```python
from build123d import *

# Parameters (mm, degrees)
SKETCH_1_W          = 50
SKETCH_1_H          = 50
EXTRUDE_1_DEPTH     = 6
SKETCH_2_W          = 6
SKETCH_2_H          = 50
EXTRUDE_2_DEPTH     = 44
SKETCH_3_R          = 10
CUT_EXTRUDE_1_DEPTH = 44
SKETCH_4_R          = 2.5
CUT_EXTRUDE_2_DEPTH = 44


with BuildPart() as part:
    # ｽｹｯﾁ1 → ﾎﾞｽ - 押し出し1 (new body)
    with BuildSketch(Plane(origin=(0, 0, 0), x_dir=(1, 0, 0), z_dir=(0, 1, 0))):
        Rectangle(SKETCH_1_W, SKETCH_1_H)
    extrude(amount=EXTRUDE_1_DEPTH)

    # ｽｹｯﾁ2 → ﾎﾞｽ - 押し出し2 (add)
    with BuildSketch(Plane(origin=(0, 6, 0), x_dir=(1, 0, 0), z_dir=(0, 1, 0))):
        with Locations((22, 0)):
            Rectangle(SKETCH_2_W, SKETCH_2_H)
    extrude(amount=EXTRUDE_2_DEPTH)

    # ｽｹｯﾁ3 → ｶｯﾄ - 押し出し1 (cut)
    with BuildSketch(Plane(origin=(25, 0, 0), x_dir=(0, 0, -1), z_dir=(1, 0, 0))):
        with Locations((0, 25)):
            Circle(SKETCH_3_R)
    extrude(amount=-CUT_EXTRUDE_1_DEPTH, mode=Mode.SUBTRACT)

    # ｽｹｯﾁ4 → ｶｯﾄ - 押し出し2 (cut)
    with BuildSketch(Plane.XZ):
        with Locations((-10.2, -15)):
            Circle(SKETCH_4_R)
        with Locations((-10.2, 15)):
            Circle(SKETCH_4_R)
    extrude(amount=-CUT_EXTRUDE_2_DEPTH, mode=Mode.SUBTRACT)


solid = part.part
```
Here's how the part is built. I have some questions about the finished solid (model axes, mm). A direction names the side the tool comes from. Coordinates: 2 decimals unless noted, no trailing zeros. Write each loop counter-clockwise with the first axis right and the second up, starting at its lowest first coordinate (ties: lowest second). Pieces come first, ordered by that corner, then holes. Notation, with made-up numbers: (16.5, 68) - (67.5, 68) arc R29 cw to (67.5, 94) - close; hole circle Ø1 at (1, 38.5). An arc over 180 degrees is marked (long way). One line per item, written item: value.
1) On a 3-axis mill with a long thin cutter (end or side, diameter ignored), from which of +Z, -Z, +X, -X, +Y, -Y can I reach the whole of each face in a straight line? I mean faces 1 (the flat face through (-3, 6, 0)), 2 (the flat face through (9, 5, -25)). Say none if no direction works.
Model answer:
face 1: +Z, -Z, -X, +Y
face 2: -Z, +X, -X, +Y, -Y
2) I'm going to push flat-ended pins straight in: P1, Ø22, axis at y = 34.5, z = 11.5, coming from the -X side; P2, Ø8, axis at x = -8, z = -11.5, coming from the +Y side. Where does each tip first touch, or does it pass through?
Model answer:
P1: stops at x = 19
P2: stops at y = 6
3) I need wall thicknesses on line 1 along Z through (x, y) = (-10.2, 2.1); line 2 along Y through (x, z) = (21, 0); line 3 along Y through (x, z) = (8.5, -21). Which ranges of each line are inside material? Lowest first, please.
Model answer:
line 1: z = -25 to -17.5, -12.5 to 12.5, 17.5 to 25
line 2: y = 0 to 15, 35 to 50
line 3: y = 0 to 6
4) Suppose I cut it at D-D on z = 15. Write out the boundary of the cut face in (x, y).
Model answer:
outline: (-25, 0) - (-12.7, 0) - (-12.7, 6) - (-25, 6) - close; (-7.7, 0) - (25, 0) - (25, 50) - (19, 50) - (19, 6) - (-7.7, 6) - close
5) Suppose I cut it at B-B on y = 25. Write out the boundary of the cut face in (x, z), and give its area (3 significant figures).
Model answer:
outline: (19, -25) - (25, -25) - (25, -10) - (19, -10) - close; (19, 10) - (25, 10) - (25, 25) - (19, 25) - close
area: 180 mm²
6) We'd pull the mould along X, two halves only. Please class faces 3 (the cylindrical face through (-12.2, 3, 13.5)), 4 (the flat face through (19, 37, 0)), 5 (the flat face through (0, 0, 0)): pulls with the +X half, pulls with the -X half, needs draft (parallel to the pull), parting line crosses it, or undercut.
Model answer:
face 3: undercut
face 4: pulls with the -X half
face 5: needs draft
7) Suppose I cut it at A-A on z = 0. Write out the boundary of the cut face in (x, y).
Model answer:
outline: (-25, 0) - (25, 0) - (25, 15) - (19, 15) - (19, 6) - (-25, 6) - close; (19, 35) - (25, 35) - (25, 50) - (19, 50) - close
8) Suppose I cut it at C-C on x = -10.2. Write out the boundary of the cut face in (y, z).
Model answer:
outline: (0, -25) - (6, -25) - (6, -17.5) - (0, -17.5) - close; (0, -12.5) - (6, -12.5) - (6, 12.5) - (0, 12.5) - close; (0, 17.5) - (6, 17.5) - (6, 25) - (0, 25) - close
